```python
from build123d import *

# Parameters (mm, degrees)
F0_W      = 127
F0_H      = 12.7
F0_W_2    = 25.4
F1_DEPTH  = 38.1
F2_W      = 6.35
F2_H      = 6.35
F3_DEPTH  = 76.2
F4_W      = 6.35
F4_H      = 14.1849974977
F4_H_2    = 13.9073220724
F5_DEPTH  = 5.08
F7_DEPTH  = 5.08
F9_DEPTH  = 119.634
F10_W     = 31.75
F10_H     = 6.35
F11_DEPTH = 5.08
F12_W     = 38.1
F12_H     = 6.4396932721
F13_DEPTH = 5.08
F14_W     = 5.08
F14_H     = 128.0755363405
F15_DEPTH = 5.08
F16_W     = 5.08
F16_H     = 128.120649606
F17_DEPTH = 5.08
F18_W     = 7.6489634812
F18_H     = 71.12
F19_DEPTH = 5.08
F20_W     = 9.6254386008
F20_H     = 73.2569846961
F21_DEPTH = 5.08


# Not quite as in the source:
# - a feature names something its author has since deleted; it is built from what else it names


with BuildPart() as f1:
    # F0 (on Right) → F1 (new body)
    with BuildSketch(Plane.YZ):
        with Locations((-23.7084774733, -8.1166389743)):
            Rectangle(F0_W, F0_H)
        with Locations((-99.9084774733, -8.1166389743)):
            Rectangle(F0_W_2, F0_H)
        with Locations((52.4915225267, -8.1166389743)):
            Rectangle(F0_W_2, F0_H)
    extrude(amount=F1_DEPTH)

    # F2 (on face) → F3 (join)
    with BuildSketch(Plane.XY.offset(-1.7666389743)):
        with Locations((3.175, 32.5670524418)):
            Rectangle(F2_W, F2_H)
        with Locations((34.925, 32.5670524418)):
            Rectangle(F2_W, F2_H)
        with Locations((3.175, -89.113903892)):
            Rectangle(F2_W, F2_H)
        with Locations((34.925, -89.113903892)):
            Rectangle(F2_W, F2_H)
    extrude(amount=F3_DEPTH)

    # F4 (on face) → F5 (join)
    with BuildSketch(Plane.YZ.offset(38.1)):
        with Locations((32.5670524418, 67.3408622769)):
            Rectangle(F4_W, F4_H)
        with Locations((-89.113903892, 67.4796999895)):
            Rectangle(F4_W, F4_H_2)
        Polygon((29.3920524418, 60.2483635281), (29.3920524418, 74.4333610257), (-28.2734257251, -1.7666389743), (-17.538718855, -1.7666389743), align=None)
        Polygon((-32.572824508, -1.7666389743), (-28.2734257251, -1.7666389743), (-85.938903892, 74.4333610257), (-85.938903892, 60.5260389533), align=None)
    extrude(amount=-F5_DEPTH)

    # F6 (on face) → F7 (join)
    with BuildSketch(Plane(origin=(0, 0, 0), x_dir=(0, -1, 0), z_dir=(-1, 0, 0))):
        Polygon((92.288903892, 59.4646334648), (92.288903892, 74.4333610257), (85.938903892, 74.4333610257), (28.2734257251, -1.7666389743), (33.4044694901, -1.7666389743), (85.938903892, 59.4646334648), align=None)
        Polygon((14.3624190241, -1.7666389743), (28.2734257251, -1.7666389743), (-29.3920524418, 74.4333610257), (-35.7420524418, 74.4333610257), (-35.7420524418, 60.1327754557), (-29.3920524418, 60.1327754557), align=None)
    extrude(amount=-F7_DEPTH)

    # F8 (on face) → F9 (cut)
    with BuildSketch(Plane.XY.offset(-1.7666389743)):
        with BuildLine():
            ThreePointArc((19.05, -20.5334774733), (16.8049359697, -25.9535415035), (22.225, -23.7084774733))
            ThreePointArc((22.225, -23.7084774733), (21.2950640303, -21.463413443), (19.05, -20.5334774733))
        make_face()
    extrude(amount=-F9_DEPTH, mode=Mode.SUBTRACT)

    # F10 (on face) → F11 (join)
    with BuildSketch(Plane.XY.offset(74.4333610257)):
        with Locations((15.875, -89.113903892)):
            Rectangle(F10_W, F10_H)
    extrude(amount=-F11_DEPTH)

    # F12 (on face) → F13 (join)
    with BuildSketch(Plane.XY.offset(74.4333610257)):
        with Locations((19.05, 32.6118990779)):
            Rectangle(F12_W, F12_H)
    extrude(amount=-F13_DEPTH)

    # F14 (on face) → F15 (join)
    with BuildSketch(Plane.XY.offset(74.4333610257)):
        with Locations((2.54, -28.2060224563)):
            Rectangle(F14_W, F14_H)
    extrude(amount=-F15_DEPTH)

    # F16 (on face) → F17 (join)
    with BuildSketch(Plane.XY.offset(74.4333610257)):
        with Locations((35.56, -28.228579089)):
            Rectangle(F16_W, F16_H)
    extrude(amount=-F17_DEPTH)

    # F18 (on face) → F19 (join)
    with BuildSketch(Plane.YZ.offset(38.1)):
        with Locations((-28.123093769, 33.7933610257)):
            Rectangle(F18_W, F18_H)
    extrude(amount=-F19_DEPTH)

    # F20 (on face) → F21 (join)
    with BuildSketch(Plane(origin=(0, 0, 0), x_dir=(0, -1, 0), z_dir=(-1, 0, 0))):
        with Locations((28.5917501897, 32.7248686777)):
            Rectangle(F20_W, F20_H)
    extrude(amount=-F21_DEPTH)


solid = f1.part
```
The model under review builds one solid part; all positions refer to its coordinate system, in mm. A direction names the side the tool comes from. Round coordinates to 2 decimals unless told otherwise and drop trailing zeros. Order: outer loops, then holes, each group sorted by start corner. A loop starts at its lowest first (then second) coordinate and runs counter-clockwise, first axis right, second up. Notation, with made-up numbers: M 87.25,-30 L 137.25,-30 A33 ccw 137.25,3 Z; hole C 49,26.25 d8. An arc over 180 degrees is marked long. Use a Markdown table: item, result.
1) Consider section D-D (y = -69.5). Write out the cut boundary in (x, z), then the cut area to 3 significant figures.
Report:
| item | result |
|---|---|
| outline | M 0,-14.47 L 38.1,-14.47 L 38.1,-1.77 L 0,-1.77 Z; M 0,40.3 L 5.08,40.3 L 5.08,52.71 L 0,52.71 Z; M 0,69.35 L 5.08,69.35 L 5.08,74.43 L 0,74.43 Z; M 33.02,41.34 L 38.1,41.34 L 38.1,52.71 L 33.02,52.71 Z; M 33.02,69.35 L 38.1,69.35 L 38.1,74.43 L 33.02,74.43 Z |
| area | 656 mm^2 |
2) Tool access review of faces 1 (the face through (36, -31.948, 36)), 2 (the face through (6.35, -89, 33)): name each direction out of +Z, -Z, +X, -X, +Y, -Y from which nothing blocks a thin tool from reaching the whole face with its end or side.
Report:
| item | result |
|---|---|
| face 1 | +X |
| face 2 | +Y, -Y |
3) Insertion check: pin 1 (3 mm diameter, centred on y = -6, z = 9, fed in from -X); pin 2 (1.5 mm diameter, centred on x = 2.5, z = 44, fed in from +Y); pin 3 (4 mm diameter, centred on x = 3.5, z = 23.5, fed in from -Y); pin 4 (2 mm diameter, centred on x = 23, y = -66.5, fed in from +Z). Each pin has a flat end and moves straight along its axis. Give the tip position at first contact, or say it passes through.
Report:
| item | result |
|---|---|
| pin 1 | x = 0 |
| pin 2 | y = 35.74 |
| pin 3 | y = -92.29 |
| pin 4 | z = -1.77 |
4) Wall thickness on line 1 along Y through (x, z) = (19, -7); line 2 along Y through (x, z) = (2.5, 57.5); line 3 along X through (y, z) = (-29.5, 3): over which ranges is each line inside the solid? List them lowest first. Write a range as [from, to].
Report:
| item | result |
|---|---|
| line 1 | [-112.61, -26.88], [-20.53, 65.19] |
| line 2 | [-92.29, -85.94], [-84.25, -73.12], [-33.4, -23.78], [16.58, 27.53], [29.39, 35.74] |
| line 3 | [0, 5.08], [33.02, 38.1] |
5) Consider section C-C (x = 36). Write out the cut boundary in (y, z).
Report:
| item | result |
|---|---|
| outline | M -112.61,-14.47 L 65.19,-14.47 L 65.19,-1.77 L 35.74,-1.77 L 35.74,69.35 L 35.83,69.35 L 35.83,74.43 L -92.29,74.43 L -92.29,-1.77 L -112.61,-1.77 Z; hole M -85.94,-1.77 L -32.57,-1.77 L -85.94,60.53 Z; hole M -82.09,69.35 L -31.95,3.09 L -31.95,69.35 Z; hole M -24.3,3.49 L 25.55,69.35 L -24.3,69.35 Z; hole M -17.54,-1.77 L 29.39,-1.77 L 29.39,60.25 Z |
6) Draft analysis for pull direction X (two halves, no side actions). For faces 3 (the face through (33.02, -29, 45)), 4 (the face through (35.596, -59.629, 29.816)), 5 (the face through (38.1, -25, 31)), state which applies: released by +X, released by -X, zero draft, split by the parting line, or undercut.
Report:
| item | result |
|---|---|
| face 3 | undercut |
| face 4 | zero draft |
| face 5 | released by +X |
7) Consider section A-A (x = 26). Write out the cut boundary in (y, z), then the cut area to 3 significant figures.
Report:
| item | result |
|---|---|
| outline | M -112.61,-14.47 L 65.19,-14.47 L 65.19,-1.77 L -112.61,-1.77 Z; M -92.29,69.35 L -85.94,69.35 L -85.94,74.43 L -92.29,74.43 Z; M 29.39,69.35 L 35.83,69.35 L 35.83,74.43 L 29.39,74.43 Z |
| area | 2,320 mm^2 |
8) Consider section B-B (y = 15.5). Write out the cut boundary in (x, z), then the cut area to 3 significant figures.
Report:
| item | result |
|---|---|
| outline | M 0,-14.47 L 38.1,-14.47 L 38.1,-1.77 L 0,-1.77 Z; M 0,40.48 L 5.08,40.48 L 5.08,56.08 L 0,56.08 Z; M 0,69.35 L 5.08,69.35 L 5.08,74.43 L 0,74.43 Z; M 33.02,41.89 L 38.1,41.89 L 38.1,56.08 L 33.02,56.08 Z; M 33.02,69.35 L 38.1,69.35 L 38.1,74.43 L 33.02,74.43 Z |
| area | 687 mm^2 |
